from build123d import *

# Parameters (mm, degrees)
ESQUISSE1_R                  = 6.1
ESQUISSE1_R_2                = 4
BOSS_EXTRU_1_DEPTH           = 10
ENL_V_MAT_EXTRU_1_DEPTH      = 12
ENL_V_MAT_EXTRU_1_DEPTH_BACK = 1


with BuildPart() as part:
    # Esquisse1 → Boss.-Extru.1 (new body)
    with BuildSketch(Plane.XY):
        Circle(ESQUISSE1_R)
        Circle(ESQUISSE1_R_2, mode=Mode.SUBTRACT)
    extrude(amount=BOSS_EXTRU_1_DEPTH)

    # Esquisse3 → Enlèv. mat.-Extru.1 (cut, two sides)
    with BuildSketch(Plane.XY) as enl_v_mat_extru_1_sk:
        with BuildLine():
            Line((-4.507231971, -3.176663454), (-4.845452386, -3.705616166))
            ThreePointArc((-4.845452386, -3.705616166), (-5.282754963, -3.05), (-5.63188393, -2.343476776))
            Line((-5.63188393, -2.343476776), (-5.004687237, -2.315045661))
            ThreePointArc((-5.004687237, -2.315045661), (-4.775431715, -2.757096786), (-4.507231971, -3.176663454))
        make_face()
        with BuildLine():
            Line((-5.409626724, -1.068770068), (-5.933750898, -1.414425779))
            ThreePointArc((-5.933750898, -1.414425779), (-6.066583562, -0.637623626), (-6.098159859, 0.149821))
            Line((-6.098159859, 0.149821), (-5.513623192, -0.079309761))
            ThreePointArc((-5.513623192, -0.079309761), (-5.483986242, -0.57639018), (-5.409626724, -1.068770068))
        make_face()
        with BuildLine():
            ThreePointArc((-4.413997755, 3.304989344), (-4.09784442, 3.689715688), (-3.748272669, 4.044351956))
            Line((-3.748272669, 4.044351956), (-3.969126703, 4.632065761))
            ThreePointArc((-3.969126703, 4.632065761), (-4.533183435, 4.081696699), (-5.021577535, 3.463200696))
            Line((-5.021577535, 3.463200696), (-4.413997755, 3.304989344))
        make_face()
        with BuildLine():
            ThreePointArc((-2.688127328, 4.814592632), (-2.242824583, 5.03746649), (-1.779231332, 5.219259201))
            Line((-1.779231332, 5.219259201), (-1.741946793, 5.845991907))
            ThreePointArc((-1.741946793, 5.845991907), (-2.481093523, 5.572627292), (-3.178828722, 5.206250854))
            Line((-3.178828722, 5.206250854), (-2.688127328, 4.814592632))
        make_face()
        with BuildLine():
            Line((0.497455265, 5.491709115), (0.786431544, 6.049092943))
            ThreePointArc((0.786431544, 6.049092943), (0, 6.1), (-0.786431544, 6.049092943))
            Line((-0.786431544, 6.049092943), (-0.497455265, 5.491709115))
            ThreePointArc((-0.497455265, 5.491709115), (0, 5.514193572), (0.497455265, 5.491709115))
        make_face()
        with BuildLine():
            Line((2.688127328, 4.814592632), (3.178828722, 5.206250854))
            ThreePointArc((3.178828722, 5.206250854), (2.481093523, 5.572627292), (1.741946793, 5.845991907))
            Line((1.741946793, 5.845991907), (1.779231332, 5.219259201))
            ThreePointArc((1.779231332, 5.219259201), (2.242824583, 5.03746649), (2.688127328, 4.814592632))
        make_face()
        with BuildLine():
            Line((3.748272669, 4.044351956), (3.969126703, 4.632065761))
            ThreePointArc((3.969126703, 4.632065761), (4.533183435, 4.081696699), (5.021577535, 3.463200696))
            Line((5.021577535, 3.463200696), (4.413997755, 3.304989344))
            ThreePointArc((4.413997755, 3.304989344), (4.09784442, 3.689715688), (3.748272669, 4.044351956))
        make_face()
        with BuildLine():
            Line((-5.069203609, 2.170139516), (-5.510008549, 2.617213364))
            ThreePointArc((-5.510008549, 2.617213364), (-5.801444749, 1.885003666), (-5.996049973, 1.121331676))
            Line((-5.996049973, 1.121331676), (-5.37664787, 1.223923373))
            ThreePointArc((-5.37664787, 1.223923373), (-5.244309729, 1.703979524), (-5.069203609, 2.170139516))
        make_face()
        with BuildLine():
            ThreePointArc((5.510008549, 2.617213364), (5.801444749, 1.885003666), (5.996049973, 1.121331676))
            Line((5.996049973, 1.121331676), (5.37664787, 1.223923373))
            ThreePointArc((5.37664787, 1.223923373), (5.244309729, 1.703979524), (5.069203609, 2.170139516))
            Line((5.069203609, 2.170139516), (5.510008549, 2.617213364))
        make_face()
        with BuildLine():
            Line((5.513623192, -0.079309761), (6.098159859, 0.149821))
            ThreePointArc((6.098159859, 0.149821), (6.066583562, -0.637623626), (5.933750898, -1.414425779))
            Line((5.933750898, -1.414425779), (5.409626724, -1.068770068))
            ThreePointArc((5.409626724, -1.068770068), (5.483986242, -0.57639018), (5.513623192, -0.079309761))
        make_face()
        with BuildLine():
            Line((5.004687237, -2.315045661), (5.63188393, -2.343476776))
            ThreePointArc((5.63188393, -2.343476776), (5.282754963, -3.05), (4.845452386, -3.705616166))
            Line((4.845452386, -3.705616166), (4.507231971, -3.176663454))
            ThreePointArc((4.507231971, -3.176663454), (4.775431715, -2.757096786), (5.004687237, -2.315045661))
        make_face()
        with BuildLine():
            ThreePointArc((3.630395391, -4.150489134), (3.24116166, -4.46107631), (2.825495864, -4.735282871))
            Line((2.825495864, -4.735282871), (2.919331138, -5.356071854))
            ThreePointArc((2.919331138, -5.356071854), (3.585490039, -4.935003666), (4.191804105, -4.431566128))
            Line((4.191804105, -4.431566128), (3.630395391, -4.150489134))
        make_face()
        with BuildLine():
            ThreePointArc((1.628375202, -5.26827533), (1.146465309, -5.393695212), (0.655205854, -5.47512886))
            Line((0.655205854, -5.47512886), (0.488431014, -6.08041406))
            ThreePointArc((0.488431014, -6.08041406), (1.268261314, -5.966700364), (2.026923269, -5.753397436))
            Line((2.026923269, -5.753397436), (1.628375202, -5.26827533))
        make_face()
        with BuildLine():
            ThreePointArc((-0.655205854, -5.47512886), (-1.146465309, -5.393695212), (-1.628375202, -5.26827533))
            Line((-1.628375202, -5.26827533), (-2.026923269, -5.753397436))
            ThreePointArc((-2.026923269, -5.753397436), (-1.268261314, -5.966700364), (-0.488431014, -6.08041406))
            Line((-0.488431014, -6.08041406), (-0.655205854, -5.47512886))
        make_face()
        with BuildLine():
            ThreePointArc((-2.919331138, -5.356071854), (-3.585490039, -4.935003666), (-4.191804105, -4.431566128))
            Line((-4.191804105, -4.431566128), (-3.630395391, -4.150489134))
            ThreePointArc((-3.630395391, -4.150489134), (-3.24116166, -4.46107631), (-2.825495864, -4.735282871))
            Line((-2.825495864, -4.735282871), (-2.919331138, -5.356071854))
        make_face()
    extrude(amount=ENL_V_MAT_EXTRU_1_DEPTH, mode=Mode.SUBTRACT)
    extrude(enl_v_mat_extru_1_sk.sketch, amount=-ENL_V_MAT_EXTRU_1_DEPTH_BACK, mode=Mode.SUBTRACT)


solid = part.part
Build history of the part. All positions in model axes, mm. A direction names the side the tool comes from. Coordinates: 2 decimals unless noted, no trailing zeros. Write each loop counter-clockwise with the first axis right and the second up, starting at its lowest first coordinate (ties: lowest second). Pieces come first, ordered by that corner, then holes.
(1) Mould opens along Y. For faces 1 (the cylindrical face through (-5.279, 3.056, 4.93)), 2 (the cylindrical face through (-4.78, -2.75, 4.93)), 3 (the cylindrical face through (1.153, -5.392, 4.93)) say: pulls with the +Y half, pulls with the -Y half, needs draft (parallel to the pull), parting line crosses it, or undercut.
(2) 3-axis set-ups, long thin cutter, end or side, ignore diameter. For faces 4 (the cylindrical face through (-1.14, -5.395, 4.93)), 5 (the cylindrical face through (-5.246, 1.697, 4.93)), 6 (the cylindrical face through (5.483, -0.583, 4.93)), 7 (the cylindrical face through (-2.49, -5.57, 4.93)), 8 (the cylindrical face through (-2.249, 5.035, 4.93)): which of +Z, -Z, +X, -X, +Y, -Y reach the whole face in a straight line?
(3) Cut at A-A on x = 1. List the corners of the cut face in (y, z), and give its area (3 significant figures).
(4) Cut at B-B on y = -0.75. List the corners of the cut face in (x, z), and give its area (3 significant figures).
(5) Pin check, flat tips, straight feed: pin 1 Ø3 at (y, z) = (2.5, 3) entering from -X; pin 2 Ø6 at (x, y) = (-0.5, -0.5) entering from +Z. Stop position of each tip, or through.
(6) Drill centre lines: line 1 (Y direction, x = 0, z = 6.75); line 2 (Y direction, x = 2.5, z = 7); line 3 (X direction, y = -1.25, z = 1.5). Where is each one in solid material? Low to high.
Working result:
1. face 1: pulls with the +Y half
1. face 2: undercut
1. face 3: pulls with the -Y half
2. face 4: +Z, -Z, -Y
2. face 5: +Z, -Z, -X
2. face 6: +Z, -Z, +X
2. face 7: +Z, -Z, -X, -Y
2. face 8: +Z, -Z, +Y
3. outline: (-5.42, 0) - (-3.87, 0) - (-3.87, 10) - (-5.42, 10) - close; (3.87, 0) - (6.02, 0) - (6.02, 10) - (3.87, 10) - close
3. area: 36.9 mm2
4. outline: (-5.46, 0) - (-3.93, 0) - (-3.93, 10) - (-5.46, 10) - close; (3.93, 0) - (5.46, 0) - (5.46, 10) - (3.93, 10) - close
4. area: 30.7 mm2
5. pin 1: stops at x = -6.02
5. pin 2: passes through
6. line 1: y = -6.1 to -4, 4 to 5.51
6. line 2: y = -5.56 to -3.12, 3.12 to 4.91
6. line 3: x = -5.68 to -3.8, 3.8 to 5.68
